```python
from build123d import *

# Parameters (mm, degrees)
SKETCH_1_R      = 20
SKETCH_1_R_2    = 16.85
EXTRUDE_1_DEPTH = 3
SKETCH_1_3_R    = 16.85
SKETCH_1_3_R_2  = 14
EXTRUDE_2_DEPTH = 7.1
SKETCH_1_4_R    = 14
SKETCH_1_4_R_2  = 8.5
EXTRUDE_3_DEPTH = 10


with BuildPart() as part:
    # 草图1 → 凸台-拉伸1 (new body)
    with BuildSketch(Plane.XY):
        Circle(SKETCH_1_R)
        Circle(SKETCH_1_R_2, mode=Mode.SUBTRACT)
    extrude(amount=EXTRUDE_1_DEPTH)

    # 草图1<3> → 凸台-拉伸2 (add)
    with BuildSketch(Plane.XY):
        Circle(SKETCH_1_3_R)
        Circle(SKETCH_1_3_R_2, mode=Mode.SUBTRACT)
    extrude(amount=EXTRUDE_2_DEPTH)

    # 草图1<4> → 凸台-拉伸3 (add)
    with BuildSketch(Plane.XY):
        Circle(SKETCH_1_4_R)
        Circle(SKETCH_1_4_R_2, mode=Mode.SUBTRACT)
    extrude(amount=EXTRUDE_3_DEPTH)


solid = part.part
```
CAD build for the part. Positions are in the model's coordinates, mm. A direction names the side the tool comes from. Round coordinates to 2 decimals unless told otherwise and drop trailing zeros. Order: outer loops, then holes, each group sorted by start corner. A loop starts at its lowest first (then second) coordinate and runs counter-clockwise, first axis right, second up.
Item 1: Probe line 1 along Y through (x, z) = (0, 5.75); line 2 along Z through (x, y) = (5.5, -14); line 3 along X through (y, z) = (-0.5, 6.5). List the from-to ranges inside material, lowest first.
Item 2: Saw through at C-C on z = 3.75. Write the cut outline in (x, y).
Item 3: Mould opens along X. For faces 3 (the face through (4.57, 7.167, 4.93)), 4 (the face through (0, -9, 10)), 5 (the face through (-2.194, 16.707, 5.021)) say: pulls with the +X half, pulls with the -X half, needs draft (parallel to the pull), parting line crosses it, or undercut.
Item 4: Saw through at A-A on x = 0. Write the cut outline in (y, z).
Item 5: Tool access for faces 1 (the face through (-6, 13, 7.1)), 2 (the face through (9, 0, 0)): list every direction of +Z, -Z, +X, -X, +Y, -Y with a clear straight run to the whole face (end or side of a thin tool).
Item 6: Pin check, flat tips, straight feed: pin 1 (5 mm diameter, centred on x = -8, z = 1, fed in from +Y); pin 2 (19.5 mm diameter, centred on x = 0, y = 0, fed in from +Z); pin 3 (2 mm diameter, centred on x = -12.5, z = 3, fed in from -Y); pin 4 (6 mm diameter, centred on x = -9, z = 4, fed in from +Y). Stop position of each tip, or through.
Item 7: Saw through at D-D on x = -9. Write the cut outline in (y, z).
Reported:
1. line 1: y = -16.85 to -8.5, 8.5 to 16.85
1. line 2: z = 0 to 7.1
1. line 3: x = -16.84 to -8.49, 8.49 to 16.84
2. outline: circle Ø33.7 at (0, 0); hole circle Ø17 at (0, 0)
3. face 3: undercut
3. face 4: needs draft
3. face 5: parting line crosses it
4. outline: (-20, 0) - (-8.5, 0) - (-8.5, 10) - (-14, 10) - (-14, 7.1) - (-16.85, 7.1) - (-16.85, 3) - (-20, 3) - close; (8.5, 0) - (20, 0) - (20, 3) - (16.85, 3) - (16.85, 7.1) - (14, 7.1) - (14, 10) - (8.5, 10) - close
5. face 1: +Z
5. face 2: -Z, +X, -X, +Y, -Y
6. pin 1: stops at y = 19.23
6. pin 2: stops at z = 10
6. pin 3: stops at y = -16.36
6. pin 4: stops at y = 19.02
7. outline: (-17.86, 0) - (17.86, 0) - (17.86, 3) - (14.25, 3) - (14.25, 7.1) - (10.72, 7.1) - (10.72, 10) - (-10.72, 10) - (-10.72, 7.1) - (-14.25, 7.1) - (-14.25, 3) - (-17.86, 3) - close
